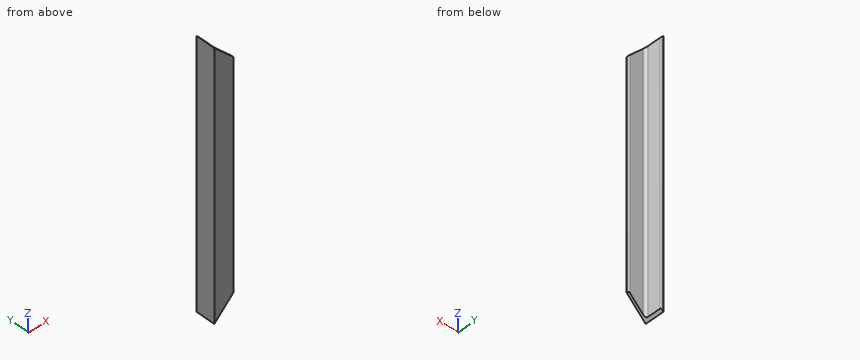
Autodesk Inventor part; units mm, degrees
ref_plane "Start Plane" through (0, 0, 100) normal (0, 0, 1) x (1, 0, 0)
ref_plane "End Plane" through (0, 0, 450) normal (0, 0, 1) x (1, 0, 0)
ref_plane "Work Plane4" through (0, 12.7, 100) normal (0.7071, 0, -0.7071) x (-0.7071, 0, -0.7071)
ref_plane "Start Plane" through (0, 0, 100) normal (0, 0, 1) x (1, 0, 0)
ref_plane "End Plane" through (0, 0, 450) normal (0, 0, 1) x (1, 0, 0)
sketch "Sketch" plane through (0, 0, 0) normal (0, 0, 1) x (1, 0, 0)
  line L0 (25.4, 0) -> (0, 0)
  line L1 (0, 0) -> (0, 25.4)
  line L2 (0, 25.4) -> (1.651, 25.4)
  line L3 (3.175, 23.876) -> (3.175, 6.477)
  line L4 (6.477, 3.175) -> (23.876, 3.175)
  line L5 (25.4, 1.651) -> (25.4, 0)
  line L6 (0, -11.0414) -> (0, 31.5385) construction
  line L7 (-11.0414, 0) -> (31.5385, 0) construction
  arc A0 (3.175, 6.477) -> (6.477, 3.175) centre (6.477, 6.477) ccw
  arc A1 (3.175, 23.876) -> (1.651, 25.4) centre (1.651, 23.876) ccw
  arc A2 (25.4, 1.651) -> (23.876, 3.175) centre (23.876, 1.651) ccw
  line L8 (0, 40.0545) -> (0, -19.5574) construction
  line L9 (-19.5574, 0) -> (40.0545, 0) construction
  point P0 (3.175, 25.4)
  point P1 (3.175, 3.175)
  point P2 (25.4, 3.175)
  dimension "d0" = 25.4
  dimension "d1" = 25.4
  dimension "d2" = 3.175
  dimension "d3" = 3.175
  dimension "d10" = 0
  dimension "d11" = 0
  dimension "d14" = 3.302
  dimension "d15" = 1.524
extrude "Body" add sketch "Sketch" along normal up to surface (350 mm away) from surface at 100
sketch "Sketch3" plane through (0, 0, 0) normal (0, 0, 1) x (1, 0, 0)
  line L0 (0, 0) -> (10, 0)
ref_plane "Work Plane3" through (0, 0, 0) normal (0, -1, 0) x (1, 0, 0)
ref_plane "Work Plane4" through (0, 12.7, 100) normal (0.7071, 0, -0.7071) x (-0.7071, 0, -0.7071)
split "Split1" plane through (0, 12.7, 100) removes the side toward (0.7071, 0, -0.7071)
ref_plane "Work Plane5" through (0, 12.7, 450) normal (0.7071, 0, 0.7071) x (0.7071, 0, -0.7071)
split "Split2" plane through (0, 12.7, 450) removes the side toward (0.7071, 0, 0.7071)
sketch "Sketch4" plane through (0, 0, 0) normal (0, -1, 0) x (1, 0, 0)
  line L0 (-2, 100) -> (12, 100)
  line L1 (-2, 450) -> (12, 450)
  dimension "d17" = 350
equation "\"d0\" = G_H"
equation "\"d1\" = G_H"
equation "\"d2\" = G_T"
equation "\"d3\" = G_T"
equation "\"d14\" = G_IR"
equation "\"d15\" = G_ER"
equation "\"d4\" = G_L"
equation "\"G_H\" = 25.4"
equation "\"G_T\" = 3.175"
equation "\"G_ER\" = 1.524"
equation "\"G_IR\" = 3.302"
equation "\"G_L\" = d17"
equation "\"ex\" = 0"
equation "\"G_OFFSET_START\" = -100"
equation "\"G_OFFSET_END\" = 0"
equation "\"d12\" = -G_OFFSET_START"
equation "\"d13\" = G_OFFSET_END + B_L"
equation "\"B_L\" = 450"
properties part number "AISC - L 1 x 1 x 1/8 - 13.78" material "Steel, Mild"
The model under review builds one solid part; all positions refer to its coordinate system, in mm. Coordinates: 2 decimals unless noted, no trailing zeros. Loops run counter-clockwise (first coordinate to the right, second up) from the corner with the lowest first, then second, coordinate; pieces in that order, holes last. Notation, with made-up numbers: M -32.75,40 L -20.75,40 A26 cw -20.75,58 Z; hole C 14.25,-15.75 d11. An arc over 180 degrees is marked long. Put each result on its own line as item: value. Start each with the question number.
Q1. Add section A-A (z = 232). Write out the cut boundary in (x, y) (3 decimals).
Q2. Wall thickness on line 1 (Y direction, x = 6.5, z = 272.5) (3 decimals); line 2 (X direction, y = 1.75, z = 399.5): over which ranges is each line inside the solid? List them lowest first.
Q3. Add section C-C (y = 15.25). Write out the cut boundary in (x, z) (3 decimals).
Q4. Clearance check with flat-ended pins moving along their axes: pin 1 (1.5 mm diameter, centred on x = 20, z = 370, fed in from +Y) (3 decimals); pin 2 (2 mm diameter, centred on y = 5.5, z = 255.5, fed in from +X); pin 3 (1.5 mm diameter, centred on x = 3, y = 9, fed in from -Z). State where each tip first meets the part, or that it passes through.
Q5. Add section B-B (x = 17). Write out the cut boundary in (y, z) (3 decimals), and give its area (3 significant figures).
Answers:
1. outline: M 0,0 L 25.4,0 L 25.4,1.651 A1.524 ccw 23.876,3.175 L 6.477,3.175 A3.302 cw 3.175,6.477 L 3.175,23.876 A1.524 ccw 1.651,25.4 L 0,25.4 Z
2. line 1: y = 0 to 3.175
2. line 2: x = 0 to 25.4
3. outline: M 0,100 L 3.175,103.175 L 3.175,446.825 L 0,450 Z
4. pin 1: stops at y = 3.175
4. pin 2: stops at x = 3.83
4. pin 3: stops at z = 102.25
5. outline: M 0,117 L 3.175,117 L 3.175,433 L 0,433 Z
5. area: 1,000 mm^2
